Solid Edge part; units mm, degrees
sketch "Sketch1" plane through (0, 0, 0) normal (0, 0, 1) x (1, 0, 0)
  circle A0 centre (0, 0) radius 4.5
  circle A1 centre (0, 0) radius 1.5
extrude "Protrusion1" add sketch "Sketch1" along normal blind 4
sketch "Sketch2" plane through (0, 0, 4) normal (0, 0, 1) x (1, 0, 0)
  circle A0 centre (0, 0) radius 2.5
  circle A1 centre (0, 0) radius 3.5
extrude "ExtrudedCutout_1" cut sketch "Sketch2" along normal mid plane 0.2526
Geometry: final body of the model. Coordinates: model frame, mm. Round coordinates to 2 decimals unless told otherwise and drop trailing zeros. Loops run counter-clockwise (first coordinate to the right, second up) from the corner with the lowest first, then second, coordinate; pieces in that order, holes last.
Q1. Section D-D on x = 3.25. Return loops of the section in (y, z).
Q2. Section C-C on z = 2.3. Return loops of the section in (x, y), plus the area to 3 significant figures.
Q3. Section A-A on y = 0. Return loops of the section in (x, z).
Q4. Pull-direction query (X, two-part tool) for faces 1 (the flat face through (0, -2, 0)), 2 (the cylindrical face through (-1.5, -0.07, 1.97)), 3 (the flat face through (2, -2, 3.874)), 4 (the cylindrical face through (-0.59, -4.46, 1.97)); classes: released by +X, released by -X, zero draft, split by the parting line, or undercut.
Q5. Pin query (flat end, axial travel): P1, Ø1.5, axis at y = -2.5, z = 0.5, coming from the +X side; P2, Ø1, axis at x = -1.5, z = 2.5, coming from the -Y side. Return the tip coordinate at first contact, or that it passes through.
Q6. Material intervals for L1, parallel to Y at x = 0, z = 0.8; L2, parallel to Y at x = -1.25, z = 2.25; L3, parallel to X at y = -1, z = 2.45, sorted ascending.
Evaluation:
1. outline: (-3.11, 0) - (3.11, 0) - (3.11, 4) - (1.3, 4) - (1.3, 3.87) - (-1.3, 3.87) - (-1.3, 4) - (-3.11, 4) - close
2. outline: circle Ø9 at (0, 0); hole circle Ø3 at (0, 0)
2. area: 56.5 mm2
3. outline: (-4.5, 0) - (-1.5, 0) - (-1.5, 4) - (-2.5, 4) - (-2.5, 3.87) - (-3.5, 3.87) - (-3.5, 4) - (-4.5, 4) - close; (1.5, 0) - (4.5, 0) - (4.5, 4) - (3.5, 4) - (3.5, 3.87) - (2.5, 3.87) - (2.5, 4) - (1.5, 4) - close
4. face 1: zero draft
4. face 2: undercut
4. face 3: undercut
4. face 4: split by the parting line
5. P1: stops at x = 4.15
5. P2: stops at y = -4.39
6. L1: y = -4.5 to -1.5, 1.5 to 4.5
6. L2: y = -4.32 to -0.83, 0.83 to 4.32
6. L3: x = -4.39 to -1.12, 1.12 to 4.39
